Can you work these out from the model? Positions are in its coordinate system, mm. Coordinates: 2 decimals unless noted, no trailing zeros. Order: outer loops, then holes, each group sorted by start corner. A loop starts at its lowest first (then second) coordinate and runs counter-clockwise, first axis right, second up. Notation, with made-up numbers: (85.5, -24) -> (116.5, -24) arc R20 cw to (116.5, -8) -> close; hole circle Ø3 at (15.25, 1.5). An arc over 180 degrees is marked (long way). Write item = value, one per line. Start each with the question number.
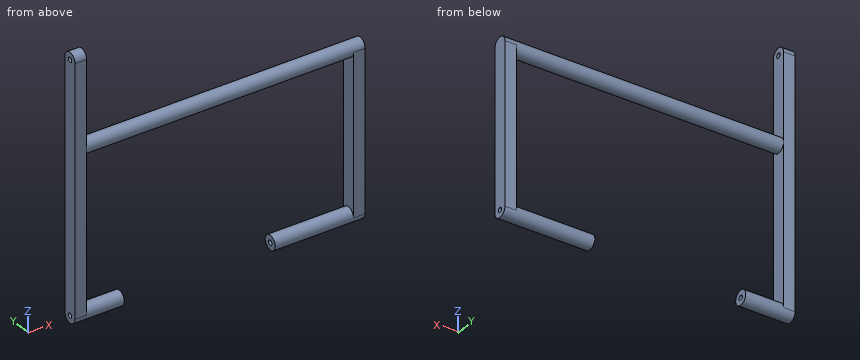
from build123d import *

# Parameters (mm, degrees)
RESSALTO_EXTRUS_O1_DEPTH   = 4
RESSALTO_EXTRUS_O2_START   = 26.96
ESBO_O2_R                  = 2.5
RESSALTO_EXTRUS_O2_DEPTH   = 26.96
RESSALTO_EXTRUS_O3_START   = 92
ESBO_O5_R                  = 2.5
RESSALTO_EXTRUS_O3_DEPTH   = 92
RESSALTO_EXTRUS_O4_START   = 4
RESSALTO_EXTRUS_O4_DEPTH   = 4
ESBO_O7_R                  = 2.5
RESSALTO_EXTRUS_O5_DEPTH   = 13
RESSALTO_EXTRUS_O6_START   = -4
RESSALTO_EXTRUS_O6_DEPTH   = 4
CORTE_EXTRUS_O1_DEPTH      = 92.502850229
CORTE_EXTRUS_O1_DEPTH_BACK = 92.502850229
ESBO_O3_R                  = 0.85
CORTE_EXTRUS_O2_DEPTH      = 117.645831473
CORTE_EXTRUS_O2_DEPTH_BACK = 117.645831473
ESBO_O4_R                  = 0.85


with BuildPart() as part:
    # Esboço1 → Ressalto-extrusão1 (new body)
    with BuildSketch(Plane(origin=(0, 0, 0), x_dir=(0, 0, -1), z_dir=(1, 0, 0))):
        with BuildLine():
            Line((-27.5, 2.5), (27.5, 2.5))
            ThreePointArc((27.5, 2.5), (30, 0), (27.5, -2.5))
            Line((27.5, -2.5), (-27.5, -2.5))
            ThreePointArc((-27.5, -2.5), (-30, 0), (-27.5, 2.5))
        make_face()
    extrude(amount=RESSALTO_EXTRUS_O1_DEPTH)

    # Esboço2 → Ressalto-extrusão2 (add)
    with BuildSketch(Plane.ZY.offset(RESSALTO_EXTRUS_O2_START)):
        with Locations((-27.5, 0)):
            Circle(ESBO_O2_R)
    extrude(amount=-RESSALTO_EXTRUS_O2_DEPTH)

    # Esboço5 → Ressalto-extrusão3 (add)
    with BuildSketch(Plane.ZY.offset(RESSALTO_EXTRUS_O3_START)):
        with Locations((27.5, 0)):
            Circle(ESBO_O5_R)
    extrude(amount=-RESSALTO_EXTRUS_O3_DEPTH)

    # Esboço6 → Ressalto-extrusão4 (add)
    with BuildSketch(Plane.ZY.offset(92).offset(RESSALTO_EXTRUS_O4_START)):
        with BuildLine():
            Line((27.5, -2.5), (-27.5, -2.5))
            ThreePointArc((-27.5, -2.5), (-30, 0), (-27.5, 2.5))
            Line((-27.5, 2.5), (27.5, 2.5))
            ThreePointArc((27.5, 2.5), (30, 0), (27.5, -2.5))
        make_face()
    extrude(amount=-RESSALTO_EXTRUS_O4_DEPTH)

    # Esboço7 → Ressalto-extrusão5 (add)
    with BuildSketch(Plane(origin=(-92, 0, 0), x_dir=(0, 0, -1), z_dir=(1, 0, 0))):
        with Locations(Location((27.5, 0, 0), (0, 0, 180))):
            Circle(ESBO_O7_R)
    extrude(amount=RESSALTO_EXTRUS_O5_DEPTH)

    # Esboço8 → Ressalto-extrusão6 (add)
    with BuildSketch(Plane(origin=(-92, 0, 0), x_dir=(0, 0, -1), z_dir=(1, 0, 0)).offset(RESSALTO_EXTRUS_O6_START)):
        with BuildLine():
            Line((-27.5, -2.5), (-57.5, -2.5))
            ThreePointArc((-57.5, -2.5), (-60, 0), (-57.5, 2.5))
            Line((-57.5, 2.5), (-27.5, 2.5))
            ThreePointArc((-27.5, 2.5), (-25, 0), (-27.5, -2.5))
        make_face()
    extrude(amount=RESSALTO_EXTRUS_O6_DEPTH)

    # Esboço3 → Corte-extrusão1 (cut, two sides: drawn at the far end of the back side and taken through both)
    with BuildSketch(Plane.ZY.offset(26.96).offset(-CORTE_EXTRUS_O1_DEPTH_BACK)):
        with Locations((-27.5, 0)):
            Circle(ESBO_O3_R)
    extrude(amount=CORTE_EXTRUS_O1_DEPTH + CORTE_EXTRUS_O1_DEPTH_BACK, mode=Mode.SUBTRACT)

    # Esboço4 → Corte-extrusão2 (cut, two sides: drawn at the far end of the back side and taken through both)
    with BuildSketch(Plane.ZY.offset(96).offset(-CORTE_EXTRUS_O2_DEPTH_BACK)):
        with Locations((57.5, 0)):
            Circle(ESBO_O4_R)
    extrude(amount=CORTE_EXTRUS_O2_DEPTH + CORTE_EXTRUS_O2_DEPTH_BACK, mode=Mode.SUBTRACT)


solid = part.part
(1) Imagine slicing it at B-B (z = 15). Write out the boundary of the cut face in (x, y).
(2) Imagine slicing it at A-A (x = -6). Write out the boundary of the cut face in (y, z).
(3) If I drill on L1, parallel to Z at x = -14, y = 0; L2, parallel to Z at x = -94.15, y = 0; L3, parallel to X at y = -1.9, z = -3.5, over which ranges is the centre line in solid material (lowest first)? Write a range as from..to.
(4) Imagine slicing it at D-D (x = -61). Write out the boundary of the cut face in (y, z), plus the area to 3 significant figures.
(5) For P1, Ø2, axis at y = 0, z = 57.5, coming from the +X side, with a flat end and sliding along its axis, tell me the tip position at first contact or that it passes through.
(6) Imagine slicing it at C-C (z = 47). Write out the boundary of the cut face in (x, y).
Result set:
q1.outline = (-96, -2.5) -> (-92, -2.5) -> (-92, 2.5) -> (-96, 2.5) -> close; (0, -2.5) -> (4, -2.5) -> (4, 2.5) -> (0, 2.5) -> close
q2.outline = circle Ø5 at (0, -27.5); circle Ø5 at (0, 27.5); hole circle Ø1.7 at (0, -27.5)
q3.L1 = -30..-28.35, -26.65..-25, 25..30
q3.L2 = -30..-28.35, -26.65..56.65, 58.35..60
q3.L3 = -96..-92, 0..4
q4.outline = circle Ø5 at (0, 27.5)
q4.area = 19.6 mm2
q5.P1 = -92
q6.outline = (-96, -2.5) -> (-92, -2.5) -> (-92, 2.5) -> (-96, 2.5) -> close
